```python
from build123d import *

# Parameters (mm, degrees)
F0_R     = 50
F1_DEPTH = 20
F2_R     = 38.5
F3_DEPTH = 25
F5_R     = 7.5
F6_DEPTH = 50
F7_R     = 15
F8_DEPTH = 10


with BuildPart() as f1:
    # F0 (on Top) → F1 (new body)
    with BuildSketch(Plane.XY):
        Circle(F0_R)
    extrude(amount=F1_DEPTH)

    # F2 (on face) → F3 (join)
    with BuildSketch(Plane.XY.offset(20)):
        Circle(F2_R)
    extrude(amount=F3_DEPTH)

    # F5 (on face) → F6 (cut)
    with BuildSketch(Plane.XY.offset(45)):
        Circle(F5_R)
    extrude(amount=-F6_DEPTH, mode=Mode.SUBTRACT)

    # F7 (on face) → F8 (cut)
    with BuildSketch(Plane(origin=(0, 0, 0), x_dir=(1, 0, 0), z_dir=(0, 0, -1))):
        Circle(F7_R)
    extrude(amount=-F8_DEPTH, mode=Mode.SUBTRACT)


solid = f1.part
```
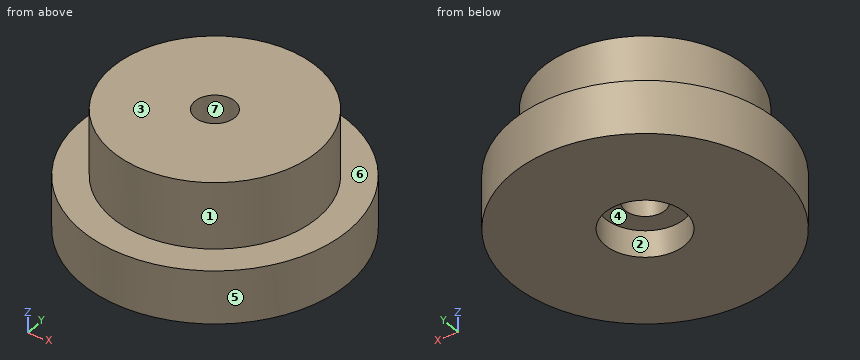
Check sheet for the modelled part. Datum: model origin and axes. Units: mm. Face numbers are marked on the shaded views. A direction names the side the tool comes from. Give positions to 0.01 mm unless a question says otherwise; leave off trailing zeros. Write each loop counter-clockwise with the first axis right and the second up, starting at its lowest first coordinate (ties: lowest second). Pieces come first, ordered by that corner, then holes.
Item 1: Scan lines: L1, parallel to Y at x = 0, z = 19; L2, parallel to Y at x = 0, z = 5; L3, parallel to Z at x = -41.5, y = 1.5. Record each from-to range of solid material in increasing order.
Item 2: Access from +Z, -Z, +X, -X, +Y, -Y to the whole of each face (thin tool, end or side, straight path). Record for the marked faces 1, 2 and 3.
Item 3: Gauge pin test, flat ends, axial feed: pin 1 (1 mm diameter, centred on y = -27.5, z = 40, fed in from +X); pin 2 (2 mm diameter, centred on y = 15, z = 17, fed in from -X); pin 3 (5 mm diameter, centred on x = -7, z = 34.5, fed in from +Y); pin 4 (12 mm diameter, centred on x = 0, y = 0, fed in from +Z) (1 decimal). Record the tip position at first contact, or that the pin passes through.
Item 4: Cross-section at A-A (x = 0). Enter the section's corners in (y, z).
Item 5: Draft check along Y on the marked faces 4, 5, 6 and 7. Enter one of: released by +Y, released by -Y, zero draft, split by the parting line, or undercut.
Item 6: Cross-section at D-D (x = 26). Enter the section's corners in (y, z).
Item 7: Cross-section at C-C (z = 32.5). Enter the section's corners in (x, y), and give its area (3 significant figures).
Report:
1. L1: y = -50 to -7.5, 7.5 to 50
1. L2: y = -50 to -15, 15 to 50
1. L3: z = 0 to 20
2. face 1: +Z
2. face 2: -Z
2. face 3: +Z, +X, -X, +Y, -Y
3. pin 1: stops at x = 27.45
3. pin 2: stops at x = -48
3. pin 3: stops at y = 38.24
3. pin 4: passes through
4. outline: (-50, 0) - (-15, 0) - (-15, 10) - (-7.5, 10) - (-7.5, 45) - (-38.5, 45) - (-38.5, 20) - (-50, 20) - close; (7.5, 10) - (15, 10) - (15, 0) - (50, 0) - (50, 20) - (38.5, 20) - (38.5, 45) - (7.5, 45) - close
5. face 4: undercut
5. face 5: split by the parting line
5. face 6: zero draft
5. face 7: undercut
6. outline: (-42.71, 0) - (42.71, 0) - (42.71, 20) - (28.39, 20) - (28.39, 45) - (-28.39, 45) - (-28.39, 20) - (-42.71, 20) - close
7. outline: circle Ø77 at (0, 0); hole circle Ø15 at (0, 0)
7. area: 4,480 mm2
